Could you check a few things on this model? Use its own coordinates, in mm. A direction names the side the tool comes from. Give positions to 0.01 mm unless a question says otherwise; leave off trailing zeros. Order: outer loops, then holes, each group sorted by start corner. A loop starts at its lowest first (then second) coordinate and runs counter-clockwise, first axis right, second up. Notation, with made-up numbers: (-9, 7) -> (1, 7) arc R14 cw to (1, 32) -> close; hole circle Ø7 at (-26.5, -31.75). An arc over 180 degrees is marked (long way). Write each question's results on one line, items separated by ' | '.
```python
from build123d import *

# Parameters (mm, degrees)
SKETCH1_W                        = 32
SKETCH1_H                        = 15
BOSS_EXTRUDE1_DEPTH              = 3
SKETCH2_R                        = 3.5
CUT_EXTRUDE1_DEPTH               = 4
M1_6X0_35_TAPPED_HOLE2_D         = 1.25
SKETCH21_R                       = 1.5
BOSS_EXTRUDE4_DEPTH              = 1
M1_6X0_35_TAPPED_HOLE3_OUTLINE_R = 0.625
M1_6X0_35_TAPPED_HOLE3_DEPTH     = 4
FILLET1_R                        = 10
M1_6X0_35_TAPPED_HOLE4_D         = 1.25
M1_6X0_35_TAPPED_HOLE4_DEPTH     = 3
M1_6X0_35_TAPPED_HOLE4_TIP       = 0.375537887


# Read off the part's stored shape, not the designer's step: M1.6x0.35 Tapped Hole3
with BuildPart() as part:
    # Sketch1 → Boss-Extrude1 (new body)
    with BuildSketch(Plane(origin=(0, 0, 0), x_dir=(1, 0, 0), z_dir=(0, 1, 0))):
        with Locations((-37.365810967, -15.175330849)):
            Rectangle(SKETCH1_W, SKETCH1_H)
    extrude(amount=BOSS_EXTRUDE1_DEPTH)

    # Sketch2 → Cut-Extrude1 (cut)
    with BuildSketch(Plane(origin=(0, 3, 0), x_dir=(1, 0, 0), z_dir=(0, 1, 0))):
        with Locations(Location((-37.365810967, -14.175330849, 0), (0, 0, 270))):
            Circle(SKETCH2_R)
    extrude(amount=-CUT_EXTRUDE1_DEPTH, mode=Mode.SUBTRACT)

    # M1.6x0.35 Tapped Hole2 (through all)
    with Locations(Plane(origin=(0, 3, 0), x_dir=(1, 0, 0), z_dir=(0, 1, 0))):
        with Locations((-34.774464311, -18.505457868), (-39.774464311, -18.505457868), (-42.274464311, -14.175330849), (-39.774464311, -9.84520383), (-34.774464311, -9.84520383), (-32.274464311, -14.175330849)):
            Hole(M1_6X0_35_TAPPED_HOLE2_D / 2)

    # Sketch21 → Boss-Extrude4 (add)
    with BuildSketch(Plane(origin=(0, 3, 0), x_dir=(1, 0, 0), z_dir=(0, 1, 0))):
        with Locations(Location((-49.774464311, -14.175330849, 0), (0, 0, 270))):
            Circle(SKETCH21_R)
        with Locations(Location((-24.774464311, -14.175330849, 0), (0, 0, 270))):
            Circle(SKETCH21_R)
    extrude(amount=BOSS_EXTRUDE4_DEPTH)

    # M1.6x0.35 Tapped Hole3 outline → M1.6x0.35 Tapped Hole3 (cut)
    with BuildSketch(Plane(origin=(0, 0, 0), x_dir=(1, 0, 0), z_dir=(0, 1, 0))):
        with Locations((-24.774464311, -14.175330849)):
            Circle(M1_6X0_35_TAPPED_HOLE3_OUTLINE_R)
        with Locations((-49.774464311, -14.175330849)):
            Circle(M1_6X0_35_TAPPED_HOLE3_OUTLINE_R)
    extrude(amount=M1_6X0_35_TAPPED_HOLE3_DEPTH, mode=Mode.SUBTRACT)

    # Fillet1
    fillet1_edges = [part.edges().sort_by_distance(p)[0] for p in [
        (-53.365810967, 1.5, 7.675330849),
        (-21.365810967, 1.5, 7.675330849),
    ]]
    fillet(fillet1_edges, radius=FILLET1_R)

    # M1.6x0.35 Tapped Hole4
    with Locations(Plane.XY.offset(22.675330849)):
        with Locations((-50.365810967, 1.5), (-24.365810967, 1.5), (-37.365810967, 1.5)):
            Hole(M1_6X0_35_TAPPED_HOLE4_D / 2, depth=M1_6X0_35_TAPPED_HOLE4_DEPTH)
            with Locations((0, 0, -(M1_6X0_35_TAPPED_HOLE4_DEPTH + M1_6X0_35_TAPPED_HOLE4_TIP / 2))):  # 118° drill point
                Cone(0, M1_6X0_35_TAPPED_HOLE4_D / 2, M1_6X0_35_TAPPED_HOLE4_TIP, mode=Mode.SUBTRACT)


solid = part.part
```
Q1. Thinking about a two-plate mould opening in Z: for faces 3 (the cylindrical face through (-40.37, 1.48, 18.32)), 4 (the flat face through (-53.366, 1, 20)), 5 (the cylindrical face through (-35.37, 1.48, 9.66)), 6 (the conical face through (-50.5, 1.4, 19.4)), which applies, +Z half, -Z half, draft (parallel to the pull), parting line (faces both ways), or undercut?
Here are the results:
face 3: undercut | face 4: draft | face 5: undercut | face 6: +Z half
Q2. I need wall thicknesses on line 1 along X through (y, z) = (1.5, 21.7); line 2 along Z through (x, y) = (-35, 1.8); line 3 along X through (y, z) = (2.7, 14.25). Which ranges of each line are inside material? Lowest first, please.
Here are the results:
line 1: x = -53.37 to -50.99, -49.74 to -37.99, -36.74 to -24.99, -23.74 to -21.37 | line 2: z = 7.68 to 9.26, 10.43 to 11.6, 16.75 to 17.92, 19.09 to 22.68 | line 3: x = -52.76 to -50.39, -49.15 to -42.89, -41.65 to -40.87, -33.87 to -32.89, -31.65 to -25.39, -24.15 to -21.97
Q3. Suppose I cut it at A-A on z = 21.25. Please give me the cut outline in (x, y) (3 decimals), and give its area (3 significant figures).
Here are the results:
outline: (-53.366, 0) -> (-21.366, 0) -> (-21.366, 3) -> (-53.366, 3) -> close; hole circle Ø1.25 at (-50.366, 1.5); hole circle Ø1.25 at (-37.366, 1.5); hole circle Ø1.25 at (-24.366, 1.5) | area: 92.3 mm²
Q4. Suppose I cut it at B-B on y = 2.5. State how many separate pieces and enclosed holes the cut face has, and give its area (3 significant figures).
Here are the results:
separate pieces: 1 | enclosed holes: 9 | area: 389 mm²
Q5. For faces 1 (the cylindrical face through (-36.74, 1.53, 21.15)), 2 (the cylindrical face through (-24.4, 1.5, 10.5)), which set-ups out of +Z, -Z, +X, -X, +Y, -Y let a thin tool reach every point of the face, with its end or its side?
Here are the results:
face 1: +Z | face 2: -Z, +X, +Y, -Y
Q6. I'm going to push flat-ended pins straight in: pin 1 Ø1 at (x, y) = (-24.37, 1.5) entering from +Z; pin 2 Ø3 at (x, z) = (-26, 19) entering from +Y. Where does each tip first touch, or does it pass through?
Here are the results:
pin 1: stops at z = 19.6 | pin 2: stops at y = 3
